Could you check a few things on this model? Use its own coordinates, in mm. A direction names the side the tool comes from. Round coordinates to 2 decimals unless told otherwise and drop trailing zeros. Write each loop counter-clockwise with the first axis right and the second up, starting at its lowest first coordinate (ties: lowest second). Pieces come first, ordered by that corner, then holes. Notation, with made-up numbers: M 62,28 L 85,28 A18 cw 85,60 Z; hole C -12,-16.75 d2. An arc over 180 degrees is marked long. One line per item, written item: value. Start each with the question number.
(1) I want a section at A-A on z = -6.75. Please give me the cut outline in (x, y) (3 decimals), and give its area (3 significant figures).
(2) I want a section at C-C on x = -133. Please give me the cut outline in (y, z) (3 decimals).
(3) Thinking about a two-plate mould opening in X: for faces 1 (the face through (-145.022, 124.471, -5.726)), 2 (the face through (-144.077, 67, -6)), 3 (the face through (-67.365, 124.422, -5.726)), which applies, released by +X, released by -X, zero draft, split by the parting line, or undercut?
(4) I'm going to push a flat-ended pin straight in: pin 1 Ø2 at (x, y) = (-106, 66) entering from -Z. Where does the tip first touch, or does it pass through?
(5) I want a section at B-B on y = 19.5. Please give me the cut outline in (x, z) (3 decimals).
(6) If I drill on L1, parallel to Y at x = -100.5, z = -3; L2, parallel to X at y = 90.5, z = -2; L3, parallel to Z at x = -90, y = 70, over which ranges is the centre line in solid material (lowest first)?
(7) Which directions (+Z, -Z, +X, -X, +Y, -Y) give clear straight access to the entire face, cutting with the end or side of a thin tool? Please do faces 4 (the face through (-107, 123.477, -6)), 5 (the face through (-67.414, 11.982, -5.726)).
(8) I want a section at D-D on y = 61.5. Please give me the cut outline in (x, z) (3 decimals), and give its area (3 significant figures).
```python
from build123d import *

# Parameters (mm, degrees)
F1_DEPTH = 9.525
F0_R     = 2.54
F2_DEPTH = 1.9
F3_R     = 2.032


with BuildPart() as f1:
    # F0 (on Top) → F1 (new body)
    with BuildSketch(Plane.XY):
        with BuildLine():
            ThreePointArc((-69.634456, 11.076584), (-67.389392, 12.00652), (-66.459456, 14.251584))
            Line((-66.459456, 14.251584), (-66.459456, 122.201584))
            ThreePointArc((-66.459456, 122.201584), (-67.389392, 124.446648), (-69.634456, 125.376584))
            Line((-69.634456, 125.376584), (-142.802102, 125.376584))
            ThreePointArc((-142.802102, 125.376584), (-145.047166, 124.446648), (-145.977102, 122.201584))
            Line((-145.977102, 122.201584), (-145.977102, 14.251584))
            ThreePointArc((-145.977102, 14.251584), (-145.047166, 12.00652), (-142.802102, 11.076584))
            Line((-142.802102, 11.076584), (-69.634456, 11.076584))
        make_face()
        with BuildLine():
            ThreePointArc((-69.634456, 123.476584), (-68.732894, 123.103146), (-68.359456, 122.201584))
            Line((-68.359456, 122.201584), (-68.359456, 14.251584))
            ThreePointArc((-68.359456, 14.251584), (-68.732894, 13.350023), (-69.634456, 12.976584))
            Line((-69.634456, 12.976584), (-142.802102, 12.976584))
            ThreePointArc((-142.802102, 12.976584), (-143.703663, 13.350023), (-144.077102, 14.251584))
            Line((-144.077102, 14.251584), (-144.077102, 122.201584))
            ThreePointArc((-144.077102, 122.201584), (-143.703663, 123.103146), (-142.802102, 123.476584))
            Line((-142.802102, 123.476584), (-69.634456, 123.476584))
        make_face(mode=Mode.SUBTRACT)
    extrude(amount=-F1_DEPTH)

    # F0 (on Top) → F2 (join)
    with BuildSketch(Plane.XY):
        with BuildLine():
            Line((-68.359456, 14.251584), (-68.359456, 122.201584))
            ThreePointArc((-68.359456, 122.201584), (-68.732894, 123.103146), (-69.634456, 123.476584))
            Line((-69.634456, 123.476584), (-142.802102, 123.476584))
            ThreePointArc((-142.802102, 123.476584), (-143.703663, 123.103146), (-144.077102, 122.201584))
            Line((-144.077102, 122.201584), (-144.077102, 14.251584))
            ThreePointArc((-144.077102, 14.251584), (-143.703663, 13.350023), (-142.802102, 12.976584))
            Line((-142.802102, 12.976584), (-69.634456, 12.976584))
            ThreePointArc((-69.634456, 12.976584), (-68.732894, 13.350023), (-68.359456, 14.251584))
        make_face()
        with Locations((-106.218279, 18.188584)):
            Circle(F0_R, mode=Mode.SUBTRACT)
        with Locations((-106.218279, 119.280584)):
            Circle(F0_R, mode=Mode.SUBTRACT)
    extrude(amount=-F2_DEPTH)

    # F3
    f3_edges = [f1.edges().sort_by_distance(p)[0] for p in [
        (-106.218279, 125.376584, 0),
    ]]
    fillet(f3_edges, radius=F3_R)


solid = f1.part
```
Found:
1. outline: M -145.977,14.252 A3.175 ccw -142.802,11.077 L -69.634,11.077 A3.175 ccw -66.459,14.252 L -66.459,122.202 A3.175 ccw -69.634,125.377 L -142.802,125.377 A3.175 ccw -145.977,122.202 Z; hole M -144.077,14.252 A1.275 ccw -142.802,12.977 L -69.634,12.977 A1.275 ccw -68.359,14.252 L -68.359,122.202 A1.275 ccw -69.634,123.477 L -142.802,123.477 A1.275 ccw -144.077,122.202 Z
1. area: 715 mm²
2. outline: M 11.077,-9.525 L 12.977,-9.525 L 12.977,-1.9 L 123.477,-1.9 L 123.477,-9.525 L 125.377,-9.525 L 125.377,-2.032 A2.032 ccw 123.345,0 L 13.109,0 A2.032 ccw 11.077,-2.032 Z
3. face 1: released by -X
3. face 2: undercut
3. face 3: released by +X
4. pin 1: stops at z = -1.9
5. outline: M -145.977,-9.525 L -144.077,-9.525 L -144.077,-1.9 L -108.394,-1.9 L -108.394,0 L -143.945,0 A2.032 ccw -145.977,-2.032 Z; M -104.043,-1.9 L -68.359,-1.9 L -68.359,-9.525 L -66.459,-9.525 L -66.459,-2.032 A2.032 ccw -68.491,0 L -104.043,0 Z
6. L1: y = 11.08 to 12.98, 123.48 to 125.38
6. L2: x = -145.98 to -144.08, -68.36 to -66.46
6. L3: z = -1.9 to 0
7. face 4: -Z
7. face 5: +Z, -Z, +X, -Y
8. outline: M -145.977,-9.525 L -144.077,-9.525 L -144.077,-1.9 L -68.359,-1.9 L -68.359,-9.525 L -66.459,-9.525 L -66.459,-2.032 A2.032 ccw -68.491,0 L -143.945,0 A2.032 ccw -145.977,-2.032 Z
8. area: 178 mm²
